The listing builds one solid part. Answer for the finished solid, in the listing's coordinates (mm). Face numbers are marked on the shaded views. A direction names the side the tool comes from. Give positions to 0.01 mm unless a question says otherwise; leave off trailing zeros. Loops run counter-clockwise (first coordinate to the right, second up) from the corner with the lowest first, then second, coordinate; pieces in that order, holes last. Notation, with made-up numbers: (70.25, -10.5) - (120.25, -10.5) arc R24 cw to (120.25, 22.5) - close; hole circle Ø2 at (88, 34.25). An arc over 180 degrees is marked (long way). One line per item, written item: value. Start each with the question number.
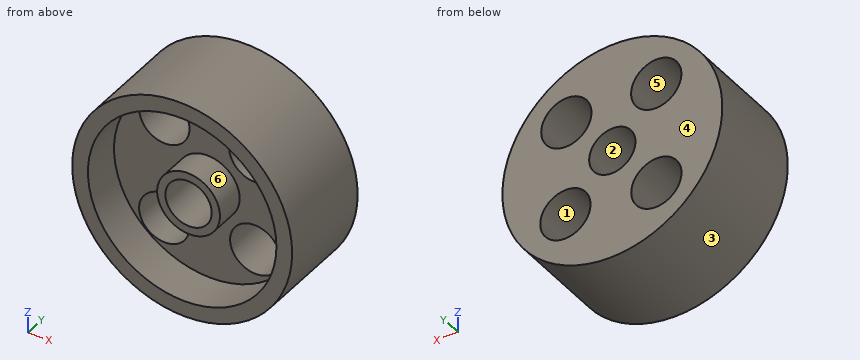
from build123d import *

# Parameters (mm, degrees)
F0_R     = 35.0012
F0_R_2   = 29.9974
F1_DEPTH = 31.242
F0_R_3   = 8.001
F0_R_4   = 9.9949
F2_DEPTH = 18.796
F0_R_5   = 7.381132
F3_DEPTH = 28.194


with BuildPart() as f1:
    # F0 (on Front) → F1 (new body)
    with BuildSketch(Plane.XZ):
        Circle(F0_R)
        Circle(F0_R_2, mode=Mode.SUBTRACT)
    extrude(amount=F1_DEPTH)

    # F0 (on Front) → F2 (join)
    with BuildSketch(Plane.XZ):
        Circle(F0_R_2)
        with Locations((-14.0208, -16.306801)):
            Circle(F0_R_3, mode=Mode.SUBTRACT)
        with Locations((14.935198, -14.7828)):
            Circle(F0_R_3, mode=Mode.SUBTRACT)
        with Locations((-13.978204, 16.333792)):
            Circle(F0_R_3, mode=Mode.SUBTRACT)
        Circle(F0_R_4, mode=Mode.SUBTRACT)
        with Locations((14.630399, 15.3924)):
            Circle(F0_R_3, mode=Mode.SUBTRACT)
    extrude(amount=F2_DEPTH)

    # F0 (on Front) → F3 (join)
    with BuildSketch(Plane.XZ):
        Circle(F0_R_4)
        Circle(F0_R_5, mode=Mode.SUBTRACT)
    extrude(amount=F3_DEPTH)


solid = f1.part
1. Flat-ended cylindrical pins translate along their axes: pin 1 (1 mm diameter, centred on y = -5.5, z = -6.5, fed in from -X); pin 2 (13 mm diameter, centred on x = 14.94, z = -14.78, fed in from +Y); pin 3 (1 mm diameter, centred on y = -25.5, z = 11.5, fed in from +X); pin 4 (3 mm diameter, centred on y = -7, z = 18, fed in from +X). Find the tip coordinate at first contact, or state that the pin passes through.
2. A cutting plane is placed at D-D (y = -13.5). Determine the outline of the cut face in (x, z), plus the area to 3 significant figures.
3. A cutting plane is placed at A-A (z = 0). Determine the outline of the cut face in (x, y).
4. A cutting plane is placed at C-C (x = -19.5). Determine the outline of the cut face in (y, z).
5. For the marked faces 5 and 6, determine the directions among +Z, -Z, +X, -X, +Y, -Y from which every point of the face is accessible in a straight line to the end or side of a thin tool.
6. A cutting plane is placed at B-B (x = 0). Determine the outline of the cut face in (y, z), plus the area to 3 significant figures.
7. Find the intervals of material crossed by L1, parallel to Z at x = 0, y = -25; L2, parallel to Z at x = 0, y = -8; L3, parallel to X at y = -16, z = -0.5, in increasing order. Write a range as [from, to].
8. Determine the mould class of the marked faces 1, 2, 3 and 4 for opening direction X: released by +X, released by -X, zero draft, split by the parting line, or undercut.
Results below:
1. pin 1: stops at x = -34.48
1. pin 2: passes through
1. pin 3: stops at x = 33.23
1. pin 4: stops at x = 30.87
2. outline: circle Ø70 at (0, 0); hole circle Ø16 at (-14.02, -16.31); hole circle Ø16 at (-13.98, 16.33); hole circle Ø14.76 at (0, 0); hole circle Ø16 at (14.63, 15.39); hole circle Ø16 at (14.94, -14.78)
2. area: 2,870 mm^2
3. outline: (-35, -31.24) - (-30, -31.24) - (-30, -18.8) - (-9.99, -18.8) - (-9.99, -28.19) - (-7.38, -28.19) - (-7.38, 0) - (-35, 0) - close; (7.38, -28.19) - (9.99, -28.19) - (9.99, -18.8) - (30, -18.8) - (30, -31.24) - (35, -31.24) - (35, 0) - (7.38, 0) - close
4. outline: (-31.24, -29.07) - (0, -29.07) - (0, -22.14) - (-18.8, -22.14) - (-18.8, -22.79) - (-31.24, -22.79) - close; (-31.24, 22.79) - (-18.8, 22.79) - (-18.8, 22.12) - (0, 22.12) - (0, 29.07) - (-31.24, 29.07) - close; (-18.8, -10.48) - (0, -10.48) - (0, 10.54) - (-18.8, 10.54) - close
5. face 5: +Y, -Y
5. face 6: -Y
6. outline: (-31.24, -35) - (0, -35) - (0, -7.38) - (-28.19, -7.38) - (-28.19, -9.99) - (-18.8, -9.99) - (-18.8, -30) - (-31.24, -30) - close; (-31.24, 30) - (-18.8, 30) - (-18.8, 9.99) - (-28.19, 9.99) - (-28.19, 7.38) - (0, 7.38) - (0, 35) - (-31.24, 35) - close
6. area: 1,210 mm^2
7. L1: z = [-35, -30], [-9.99, -7.38], [7.38, 9.99], [30, 35]
7. L2: z = [-35, -7.38], [7.38, 35]
7. L3: x = [-35, -7.36], [7.36, 35]
8. face 1: undercut
8. face 2: undercut
8. face 3: split by the parting line
8. face 4: zero draft
